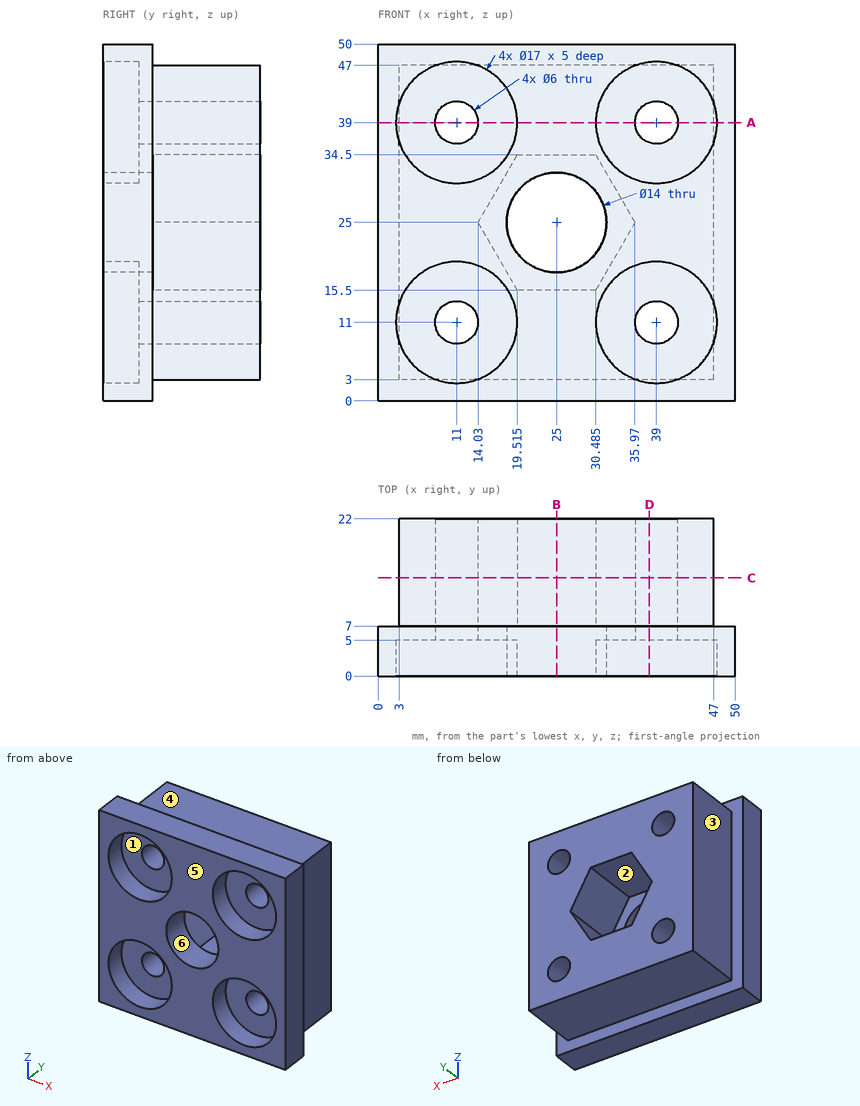
Check sheet for the drawn part. Datum: minimum x, y, z corner. Units: mm. A direction names the side the tool comes from. Round coordinates to 2 decimals unless told otherwise and drop trailing zeros. Loops run counter-clockwise (first coordinate to the right, second up) from the corner with the lowest first, then second, coordinate; pieces in that order, holes last.
Item 1: Thickness scan on line 1 (Z direction, x = 11, y = 18.25); line 2 (Z direction, x = 25, y = 5.25); line 3 (Z direction, x = 37, y = 17.5) (1 decimal). Record the ranges inside material, lowest first.
Item 2: Access from +Z, -Z, +X, -X, +Y, -Y to the whole of each face (thin tool, end or side, straight path). Record for the marked faces 1, 2 and 3.
Item 3: Cross-section at A-A on z = 39. Record the boundary of the cut face in (x, y), then the cut area to 3 significant figures.
Item 4: Gauge pin test, flat ends, axial feed: pin 1 (10 mm diameter, centred on x = 39, z = 39, fed in from -Y); pin 2 (4.5 mm diameter, centred on y = 15.5, z = 22, fed in from +X); pin 3 (8.5 mm diameter, centred on x = 13.5, z = 14.5, fed in from -Y); pin 4 (9 mm diameter, centred on x = 27, y = 17, fed in from -Z). Record the tip position at first contact, or that the pin passes through.
Item 5: Cross-section at B-B on x = 25. Record the boundary of the cut face in (y, z).
Item 6: Cross-section at C-C on y = 13.75. Record the boundary of the cut face in (x, z) (1 decimal).
Item 7: Cross-section at D-D on x = 38. Record the boundary of the cut face in (y, z).
Item 8: Mould release check, pull along Z, two halves, no side actions. Record for the marked faces 4, 5 and 6: pulls with the +Z half, pulls with the -Z half, needs draft (parallel to the pull), parting line crosses it, or undercut.
Answer sheet:
1. line 1: z = 3 to 8, 14 to 36, 42 to 47
1. line 2: z = 0 to 18, 32 to 50
1. line 3: z = 3 to 8.8, 13.2 to 36.8, 41.2 to 47
2. face 1: -Y
2. face 2: +Y
2. face 3: +Z, -Z, -X, +Y
3. outline: (0, 0) - (2.5, 0) - (2.5, 5) - (8, 5) - (8, 22) - (3, 22) - (3, 7) - (0, 7) - close; (14, 5) - (19.5, 5) - (19.5, 0) - (30.5, 0) - (30.5, 5) - (36, 5) - (36, 22) - (14, 22) - close; (42, 5) - (47.5, 5) - (47.5, 0) - (50, 0) - (50, 7) - (47, 7) - (47, 22) - (42, 22) - close
3. area: 636 mm2
4. pin 1: stops at y = 5
4. pin 2: stops at x = 47
4. pin 3: stops at y = 0
4. pin 4: stops at z = 3
5. outline: (0, 0) - (7, 0) - (7, 3) - (22, 3) - (22, 15.5) - (7, 15.5) - (7, 18) - (0, 18) - close; (0, 32) - (7, 32) - (7, 34.5) - (22, 34.5) - (22, 47) - (7, 47) - (7, 50) - (0, 50) - close
6. outline: (3, 3) - (47, 3) - (47, 47) - (3, 47) - close; hole circle Ø6 at (11, 11); hole circle Ø6 at (11, 39); hole (14, 25) - (19.5, 15.5) - (30.5, 15.5) - (36, 25) - (30.5, 34.5) - (19.5, 34.5) - close; hole circle Ø6 at (39, 11); hole circle Ø6 at (39, 39)
7. outline: (0, 0) - (7, 0) - (7, 3) - (22, 3) - (22, 8.17) - (5, 8.17) - (5, 2.56) - (0, 2.56) - close; (0, 19.44) - (5, 19.44) - (5, 13.83) - (22, 13.83) - (22, 36.17) - (5, 36.17) - (5, 30.56) - (0, 30.56) - close; (0, 47.44) - (5, 47.44) - (5, 41.83) - (22, 41.83) - (22, 47) - (7, 47) - (7, 50) - (0, 50) - close
8. face 4: pulls with the +Z half
8. face 5: needs draft
8. face 6: undercut
